Autodesk Inventor part; units mm, degrees
ref_plane "YZ Plane" through (0, 0, 0) normal (1, 0, 0) x (0, 1, 0)
ref_plane "XZ Plane" through (0, 0, 0) normal (0, 1, 0) x (-1, 0, 0)
ref_plane "XY Plane" through (0, 0, 0) normal (0, 0, 1) x (1, 0, 0)
sketch "Sketch1" plane through (0, 0, 0) normal (0, 1, 0) x (-1, 0, 0)
  circle A0 centre (0, 0) radius 160
  circle A1 centre (0, 0) radius 325
  line L0 (0, 0) -> (0, -325)
  line L1 (0, 0) -> (-229.8097, -229.8097)
  line L2 (0, 0) -> (28.3256, -323.7633)
  line L3 (0, 0) -> (-208.906, -248.9644)
  circle A2 centre (0, 0) radius 285
  circle A3 centre (0, 0) radius 265
  circle A4 centre (0, 0) radius 200
  circle A5 centre (0, 0) radius 220
  line L4 (0, -220) -> (17.4311, -199.2389)
  line L5 (0, -265) -> (24.8394, -283.9155)
  line L6 (-128.5575, -153.2089) -> (-155.5635, -155.5635)
  line L7 (-187.3833, -187.3833) -> (-183.1945, -218.3227)
  point P0 (-113.1371, -113.1371)
  point P1 (0, -160)
  dimension "d0" = 650
  dimension "d1" = 320
  dimension "d2" = 45
  dimension "d13" = 40
  dimension "d14" = 40
  dimension "d15" = 20
  dimension "d16" = 20
  dimension "d17" = 5
  dimension "d18" = 5
extrude "Extrusion1" add sketch "Sketch1" along normal blind 5 contours A0 L3 A4 L1 | A0 L0 A4 L3 | A4 L6 L1 | L2 A5 L4 | A4 L0 A5 L3 | L2 A3 L0 A5 | L0 A3 L3 A5 | L7 A2 L1 | L2 L5 A3 | L0 A2 L3 A3 | A2 L3 A1 L1 | A2 L0 A1 L3
sketch "Sketch2" plane through (0, 5, 0) normal (0, 1, 0) x (1, 0, 0)
  arc A0 (229.8097, 229.8097) -> (0, 325) centre (0, 0) ccw
  line L0 (0, 325) -> (0, 265)
  arc A1 (113.1371, 113.1371) -> (0, 160) centre (0, 0) ccw
  line L1 (113.1371, 113.1371) -> (155.5635, 155.5635)
  circle A2 centre (0, 0) radius 190
  circle A3 centre (0, 0) radius 210
  line L2 (155.5635, 155.5635) -> (128.5575, 153.2089)
  line L3 (128.5575, 153.2089) -> (183.1945, 218.3227)
  line L4 (183.1945, 218.3227) -> (187.3833, 187.3833)
  line L5 (187.3833, 187.3833) -> (229.8097, 229.8097)
  line L6 (0, 265) -> (-24.8394, 283.9155)
  line L7 (-24.8394, 283.9155) -> (-17.4311, 199.2389)
  line L8 (-17.4311, 199.2389) -> (0, 220)
  line L9 (0, 220) -> (0, 160)
  point P0 (148.4924, 148.4924)
  point P1 (0, 210)
  point P2 (0, 190)
  point P3 (134.3503, 134.3503)
  point P4 (0, 190)
  point P5 (0, 210)
  point P6 (-8.542, 209.8262)
  point P7 (-18.3027, 209.2009)
  point P8 (142.3294, 154.4096)
  point P9 (134.9854, 160.8693)
  dimension "d5" = 420
  dimension "d6" = 20
extrude "Extrusion2" add sketch "Sketch2" along normal blind 62 contours L3 L2 A3 L1 A2 L9 | A3 L2 L3
sketch "Sketch3" plane through (0, 67, 0) normal (0, 1, 0) x (1, 0, 0)
  line L0 (134.3503, 134.3503) -> (148.4924, 148.4924)
  arc A0 (148.4924, 148.4924) -> (0, 210) centre (0, 0) ccw
  circle A1 centre (0, 0) radius 190
  circle A2 centre (0, 0) radius 249
  line L1 (0, 190) -> (0, 160)
  line L2 (113.1371, 113.1371) -> (134.3503, 134.3503)
  arc A3 (148.4924, 148.4924) -> (142.3294, 154.4096) centre (0, 0) ccw
  line L3 (148.4924, 148.4924) -> (155.5635, 155.5635)
  arc A4 (229.8097, 229.8097) -> (0, 325) centre (0, 0) ccw
  line L4 (0, 220) -> (0, 210)
  line L5 (-17.4311, 199.2389) -> (0, 220)
  line L6 (0, 325) -> (0, 265)
  arc A5 (134.9854, 160.8693) -> (0, 210) centre (0, 0) ccw
  line L7 (134.9854, 160.8693) -> (183.1945, 218.3227)
  line L8 (183.1945, 218.3227) -> (187.3833, 187.3833)
  line L9 (0, 265) -> (-24.8394, 283.9155)
  line L10 (-24.8394, 283.9155) -> (-17.4311, 199.2389)
  arc A6 (148.4924, 148.4924) -> (142.3294, 154.4096) centre (0, 0) ccw
  line L11 (-17.4311, 199.2389) -> (0, 220)
  arc A7 (134.9854, 160.8693) -> (0, 210) centre (0, 0) ccw
  line L12 (134.9854, 160.8693) -> (183.1945, 218.3227)
  line L13 (183.1945, 218.3227) -> (187.3833, 187.3833)
  arc A8 (229.8097, 229.8097) -> (0, 325) centre (0, 0) ccw
  line L14 (0, 325) -> (0, 265)
  line L15 (0, 265) -> (-24.8394, 283.9155)
  line L16 (-24.8394, 283.9155) -> (-17.4311, 199.2389)
  line L17 (187.3833, 187.3833) -> (229.8097, 229.8097)
  arc A9 (134.3503, 134.3503) -> (0, 190) centre (0, 0) ccw
  line L18 (0, 190) -> (0, 160)
  arc A10 (113.1371, 113.1371) -> (0, 160) centre (0, 0) ccw
  line L19 (113.1371, 113.1371) -> (134.3503, 134.3503)
  line L20 (155.5635, 155.5635) -> (142.3294, 154.4096)
  line L21 (187.3833, 187.3833) -> (229.8097, 229.8097)
  line L22 (0, 220) -> (0, 210)
  arc A11 (134.3503, 134.3503) -> (0, 190) centre (0, 0) ccw
  arc A12 (113.1371, 113.1371) -> (0, 160) centre (0, 0) ccw
  line L23 (148.4924, 148.4924) -> (155.5635, 155.5635)
  line L24 (155.5635, 155.5635) -> (142.3294, 154.4096)
  arc A13 (134.3503, 134.3503) -> (0, 190) centre (0, 0) ccw
  line L25 (0, 210) -> (0, 190)
  line L26 (0, 0) -> (229.8097, 229.8097)
  arc A14 (229.8097, 229.8097) -> (0, 325) centre (0, 0) ccw
  line L27 (0, 0) -> (0, 325)
  point P0 (176.0696, 176.0696)
  point P1 (0, 249)
  point P2 (-18.3027, 209.2009)
  point P3 (-21.7018, 248.0525)
  point P4 (160.0541, 190.7451)
  point P5 (0, 210)
  point P6 (-8.542, 209.8262)
  point P7 (0, 210)
  point P8 (0, 210)
  point P9 (176.0696, 176.0696)
  point P10 (0, 249)
  dimension "d12" = 59
extrude "Extrusion3" add sketch "Sketch3" along normal blind 10 contours A1 L25 A0 L0 | A0 L20 L3 | A0 L7 A2 L26 L20 | L4 L27 A2 L7 A0
sketch "Sketch5" plane through (0, 5, 0) normal (0, 1, 0) x (1, 0, 0)
  circle A0 centre (0, 0) radius 295
  arc A1 (134.9854, 160.8693) -> (0, 210) centre (0, 0) ccw
  line L0 (134.9854, 160.8693) -> (183.1945, 218.3227)
  line L1 (183.1945, 218.3227) -> (187.3833, 187.3833)
  line L2 (187.3833, 187.3833) -> (229.8097, 229.8097)
  arc A2 (229.8097, 229.8097) -> (0, 325) centre (0, 0) ccw
  line L3 (0, 325) -> (0, 265)
  line L4 (0, 265) -> (-24.8394, 283.9155)
  line L5 (-24.8394, 283.9155) -> (-17.4311, 199.2389)
  line L6 (-17.4311, 199.2389) -> (0, 220)
  line L7 (0, 220) -> (0, 210)
  point P0 (40.9671, 292.1416)
  point P1 (167.4373, 242.878)
  point P2 (105.8364, 275.361)
  dimension "d26" = 30
hole "Hole1" at (40.9671, 5, -292.1416) at (167.4373, 5, -242.878) at (105.8364, 5, -275.361) direction (0, -1, 0) diameter 1.7551 end through all
properties part number "Carousel Base Plate v2"
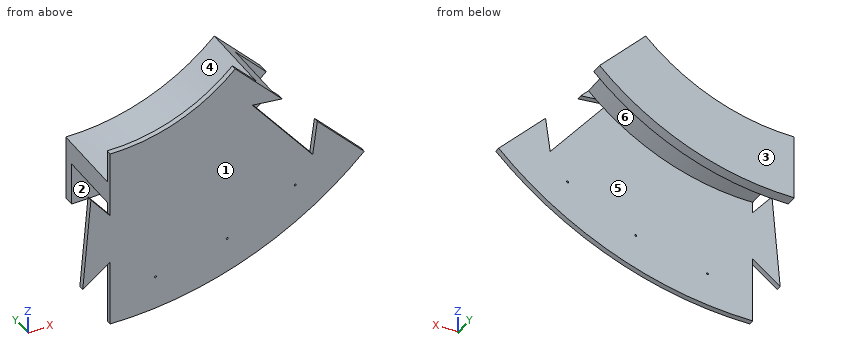
Could you check a few things on this model? Use its own coordinates, in mm. Face numbers are marked on the shaded views. A direction names the side the tool comes from. Round coordinates to 2 decimals unless told otherwise and drop trailing zeros. Order: outer loops, then holes, each group sorted by start corner. A loop starts at its lowest first (then second) coordinate and runs counter-clockwise, first axis right, second up.
(1) Please list where these lines run through material, in increasing order: line 1 along Y through (x, z) = (11, -227.5); line 2 along Y through (x, z) = (38, -282.5); line 3 along Z through (x, y) = (26, 51).
Response values:
line 1: y = 0 to 5, 67 to 77
line 2: y = 0 to 5
line 3: z = -208.38 to -188.21
(2) If we mould it in two halves opening along Y, with no side actions, what happens to the marked faces 3, 4, 5 and 6? For each: released by +Y, released by -Y, zero draft, split by the parting line, or undercut.
Response values:
face 3: released by +Y
face 4: zero draft
face 5: undercut
face 6: undercut
(3) I'm going to push flat-ended pins straight in: pin 1 (4 mm diameter, centred on x = 89, y = 42.5, fed in from -Z); pin 2 (1 mm diameter, centred on y = 28, z = -156.5, fed in from +X); pin 3 (1.1 mm diameter, centred on x = 40.97, z = -292.14, fed in from -Y); pin 4 (6 mm diameter, centred on x = 40, z = -189, fed in from -Y). Where does each tip first touch, or does it pass through?
Response values:
pin 1: stops at z = -191.13
pin 2: stops at x = 140.58
pin 3: passes through
pin 4: stops at y = 0
(4) Which directions (+Z, -Z, +X, -X, +Y, -Y) give clear straight access to the entire face, cutting with the end or side of a thin tool? Please do the marked faces 1 and 2.
Response values:
face 1: +Z, -Z, +X, -X, -Y
face 2: -Z, +X
(5) Imagine slicing it at B-B (z = -215). Write out the boundary of the cut face in (x, y).
Response values:
outline: (-18.81, 0) - (-4.2, 0) - (-4.2, 5) - (-18.81, 5) - close; (0, 0) - (180.41, 0) - (180.41, 5) - (0, 5) - close; (0, 67) - (125.6, 67) - (125.6, 77) - (0, 77) - close; (183.64, 0) - (215, 0) - (215, 5) - (183.64, 5) - close
(6) Imagine slicing it at D-D (x = 48). Write out the boundary of the cut face in (y, z).
Response values:
outline: (0, -321.44) - (5, -321.44) - (5, -204.44) - (67, -204.44) - (67, -244.33) - (77, -244.33) - (77, -183.84) - (5, -183.84) - (5, -152.63) - (0, -152.63) - close
(7) Imagine slicing it at C-C (y = 15.5). Write out the boundary of the cut face in (x, z), plus the area to 3 significant figures.
Response values:
outline: (0, -210) arc R210 ccw to (148.49, -148.49) - (134.35, -134.35) arc R190 cw to (0, -190) - close
area: 3,140 mm2
(8) Imagine slicing it at A-A (x = 161). Write out the boundary of the cut face in (y, z).
Response values:
outline: (0, -282.32) - (5, -282.32) - (5, -191.87) - (0, -191.87) - close; (67, -189.95) - (77, -189.95) - (77, -161) - (67, -161) - close
